Verification items for the finished model (mm, model axes). Face numbers are marked on the shaded views. A direction names the side the tool comes from. Give positions to 0.01 mm unless a question says otherwise; leave off trailing zeros. Write each loop counter-clockwise with the first axis right and the second up, starting at its lowest first coordinate (ties: lowest second). Pieces come first, ordered by that corner, then holes. Notation, with made-up numbers: (80, -31) - (103, -31) arc R22 ccw to (103, -18) - close; hole circle Ø2 at (-8, -28.5). An arc over 180 degrees is marked (long way). Answer as a JSON object with one key per item and string values. Group by question number.
Item 1: Go/stop test with flat-tipped pins: pin 1 (3.5 mm diameter, centred on x = 54.05, y = -5.05, fed in from +Z); pin 2 (10.5 mm diameter, centred on y = -10, z = 16.43, fed in from -X); pin 3 (1.6 mm diameter, centred on y = -3, z = 16.43, fed in from -X); pin 4 (1.2 mm diameter, centred on y = -17.5, z = 8.93, fed in from +X). Record where each tip stops, or that it passes through.
Item 2: Scan lines: line 1 along Y through (x, z) = (44.15, -0.65); line 2 along X through (y, z) = (-1.75, 16.5); line 3 along Z through (x, y) = (72.15, -17.5). Record each from-to range of solid material in increasing order. Write a range as [from, to].
Item 3: Draft check along X on the marked faces 1, 2 and 3. Enter one of: +X half, -X half, draft (parallel to the pull), parting line (faces both ways), or undercut.
Item 4: Sectioned sample at B-B, the plane z = 11. Record the boundary of the cut face in (x, y), and give its area (3 significant figures).
Item 5: Sectioned sample at A-A, the plane x = 54.05. Record the boundary of the cut face in (y, z), and give its area (3 significant figures).
Item 6: Sectioned sample at C-C, the plane y = -5.05. Record the boundary of the cut face in (x, z), and give its area (3 significant figures).
Item 7: Tool access check on the marked faces 4 and 5. Record the directions out of +Z, -Z, +X, -X, +Y, -Y that give a thin tool (end or side, any length) a straight path to the whole face; none if there is none.
Item 8: Sectioned sample at D-D, the plane y = -8. Record the boundary of the cut face in (x, z).
```python
from build123d import *

# Parameters (mm, degrees)
IZIM1_R                      = 4
IZIM1_R_2                    = 1
IZIM1_R_3                    = 3
IZIM1_R_4                    = 1.5
TABAN_FLAN_2_DEPTH           = 2
IZGIDEN_START                = -1
IZGIDEN_B_KME2_OUTLINE_W     = 20
IZGIDEN_B_KME2_OUTLINE_H     = 2
IZGIDEN_B_KME2_DEPTH         = 26.570796327
IZGIDEN_START_2              = 72.629203673
IZGIDEN_B_KME2_2_OUTLINE_W   = 20
IZGIDEN_B_KME2_2_OUTLINE_H   = 2
IZGIDEN_B_KME2_2_DEPTH       = 25.570796327
IZGIDEN_START_3              = 25.570796327
IZGIDEN_B_KME2_3_OUTLINE_R   = 1
IZGIDEN_B_KME2_3_OUTLINE_R_2 = 4
IZGIDEN_B_KME2_3_DEPTH       = 3
IZGIDEN_START_4              = 69.629203673
IZGIDEN_B_KME2_4_OUTLINE_R   = 1
IZGIDEN_B_KME2_4_OUTLINE_R_2 = 4
IZGIDEN_B_KME2_4_DEPTH       = 3
IZGIDEN_START_5              = 70.629203673
IZGIDEN_B_KME2_5_OUTLINE_R   = 1
IZGIDEN_B_KME2_5_DEPTH       = 2
IZGIDEN_B_KME2_6_OUTLINE_R   = 1
IZGIDEN_B_KME2_6_DEPTH       = 2
IZGIDEN_START_6              = -21
IZGIDEN_B_KME2_7_DEPTH       = 22


with BuildPart() as part:
    # Taban-Flanş2: sheet metal written as solids
    # Çizim1 → Taban-Flanş2 (new body)
    with BuildSketch(Plane.XY):
        with BuildLine():
            Line((98.2, -3), (98.2, -17))
            ThreePointArc((98.2, -17), (97.321320344, -19.121320344), (95.2, -20))
            Line((95.2, -20), (10, -20))
            ThreePointArc((10, -20), (0, -10), (10, 0))
            Line((10, 0), (95.2, 0))
            ThreePointArc((95.2, 0), (97.321320344, -0.878679656), (98.2, -3))
        make_face()
        with Locations((10, -10)):
            Circle(IZIM1_R, mode=Mode.SUBTRACT)
        with Locations((10, -17)):
            Circle(IZIM1_R_2, mode=Mode.SUBTRACT)
        with Locations((3, -10)):
            Circle(IZIM1_R_2, mode=Mode.SUBTRACT)
        with Locations((10, -3)):
            Circle(IZIM1_R_2, mode=Mode.SUBTRACT)
        with Locations((17, -10)):
            Circle(IZIM1_R_2, mode=Mode.SUBTRACT)
        with Locations((88.2, -10)):
            Circle(IZIM1_R, mode=Mode.SUBTRACT)
        with Locations((80.7, -2.5)):
            Circle(IZIM1_R_2, mode=Mode.SUBTRACT)
        with Locations((95.7, -2.5)):
            Circle(IZIM1_R_2, mode=Mode.SUBTRACT)
        with Locations((95.7, -17.5)):
            Circle(IZIM1_R_2, mode=Mode.SUBTRACT)
        with Locations((80.7, -17.5)):
            Circle(IZIM1_R_2, mode=Mode.SUBTRACT)
        with Locations((49.1, -10)):
            Circle(IZIM1_R_3, mode=Mode.SUBTRACT)
        with Locations((54.05, -5.05)):
            Circle(IZIM1_R_4, mode=Mode.SUBTRACT)
        with Locations((44.15, -5.05)):
            Circle(IZIM1_R_4, mode=Mode.SUBTRACT)
        with Locations((44.15, -14.95)):
            Circle(IZIM1_R_4, mode=Mode.SUBTRACT)
        with Locations((54.05, -14.95)):
            Circle(IZIM1_R_4, mode=Mode.SUBTRACT)
    extrude(amount=-TABAN_FLAN_2_DEPTH)

    # Çizgiden Bükme2: read off the stored shape, not the designer's step
    # Çizgiden Bükme2 outline → Çizgiden Bükme2 (cut)
    with BuildSketch(Plane.YZ.offset(IZGIDEN_START)):
        with Locations((-10, -1)):
            Rectangle(IZGIDEN_B_KME2_OUTLINE_W, IZGIDEN_B_KME2_OUTLINE_H)
    extrude(amount=IZGIDEN_B_KME2_DEPTH, mode=Mode.SUBTRACT)

    # izgiden B_kme2 2 outline → izgiden B_kme2 2 (cut)
    with BuildSketch(Plane.YZ.offset(IZGIDEN_START_2)):
        with Locations((-10, -1)):
            Rectangle(IZGIDEN_B_KME2_2_OUTLINE_W, IZGIDEN_B_KME2_2_OUTLINE_H)
    extrude(amount=IZGIDEN_B_KME2_2_DEPTH, mode=Mode.SUBTRACT)

    # izgiden B_kme2 3 outline → izgiden B_kme2 3 (add)
    with BuildSketch(Plane.YZ.offset(IZGIDEN_START_3)):
        with BuildLine():
            Line((-20, 0), (0, 0))
            Line((0, 0), (0, 16.429203673))
            ThreePointArc((0, 16.429203673), (-0.620384974, 19.896597791), (-2.404564394, 22.933768067))
            ThreePointArc((-2.404564394, 22.933768067), (-3.207106781, 23.222096892), (-3.495435606, 24.024639279))
            ThreePointArc((-3.495435606, 24.024639279), (-10, 26.429203673), (-16.504564394, 24.024639279))
            ThreePointArc((-16.504564394, 24.024639279), (-16.792893219, 23.222096892), (-17.595435606, 22.933768067))
            ThreePointArc((-17.595435606, 22.933768067), (-19.379615026, 19.896597791), (-20, 16.429203673))
            Line((-20, 16.429203673), (-20, 0))
        make_face()
        with Locations((-17.5, 8.929203673)):
            Circle(IZGIDEN_B_KME2_3_OUTLINE_R, mode=Mode.SUBTRACT)
        with Locations((-10, 9.429203673)):
            Circle(IZGIDEN_B_KME2_3_OUTLINE_R, mode=Mode.SUBTRACT)
        with Locations((-2.5, 8.929203673)):
            Circle(IZGIDEN_B_KME2_3_OUTLINE_R, mode=Mode.SUBTRACT)
        with Locations((-17, 16.429203673)):
            Circle(IZGIDEN_B_KME2_3_OUTLINE_R, mode=Mode.SUBTRACT)
        with Locations((-10, 16.429203673)):
            Circle(IZGIDEN_B_KME2_3_OUTLINE_R_2, mode=Mode.SUBTRACT)
        with Locations((-3, 16.429203673)):
            Circle(IZGIDEN_B_KME2_3_OUTLINE_R, mode=Mode.SUBTRACT)
        with Locations((-10, 23.429203673)):
            Circle(IZGIDEN_B_KME2_3_OUTLINE_R, mode=Mode.SUBTRACT)
    extrude(amount=IZGIDEN_B_KME2_3_DEPTH)

    # izgiden B_kme2 4 outline → izgiden B_kme2 4 (add)
    with BuildSketch(Plane.YZ.offset(IZGIDEN_START_4)):
        with BuildLine():
            Line((-20, 0), (0, 0))
            Line((0, 0), (0, 16.429203673))
            ThreePointArc((0, 16.429203673), (-0.620384974, 19.896597791), (-2.404564394, 22.933768067))
            ThreePointArc((-2.404564394, 22.933768067), (-3.207106781, 23.222096892), (-3.495435606, 24.024639279))
            ThreePointArc((-3.495435606, 24.024639279), (-10, 26.429203673), (-16.504564394, 24.024639279))
            ThreePointArc((-16.504564394, 24.024639279), (-16.792893219, 23.222096892), (-17.595435606, 22.933768067))
            ThreePointArc((-17.595435606, 22.933768067), (-19.379615026, 19.896597791), (-20, 16.429203673))
            Line((-20, 16.429203673), (-20, 0))
        make_face()
        with Locations((-17.5, 8.929203673)):
            Circle(IZGIDEN_B_KME2_4_OUTLINE_R, mode=Mode.SUBTRACT)
        with Locations((-10, 9.429203673)):
            Circle(IZGIDEN_B_KME2_4_OUTLINE_R, mode=Mode.SUBTRACT)
        with Locations((-2.5, 8.929203673)):
            Circle(IZGIDEN_B_KME2_4_OUTLINE_R, mode=Mode.SUBTRACT)
        with Locations((-17, 16.429203673)):
            Circle(IZGIDEN_B_KME2_4_OUTLINE_R, mode=Mode.SUBTRACT)
        with Locations((-10, 16.429203673)):
            Circle(IZGIDEN_B_KME2_4_OUTLINE_R_2, mode=Mode.SUBTRACT)
        with Locations((-3, 16.429203673)):
            Circle(IZGIDEN_B_KME2_4_OUTLINE_R, mode=Mode.SUBTRACT)
        with Locations((-10, 23.429203673)):
            Circle(IZGIDEN_B_KME2_4_OUTLINE_R, mode=Mode.SUBTRACT)
    extrude(amount=IZGIDEN_B_KME2_4_DEPTH)

    # izgiden B_kme2 5 outline → izgiden B_kme2 5 (add)
    with BuildSketch(Plane.YZ.offset(IZGIDEN_START_5)):
        with BuildLine():
            ThreePointArc((-2.404564394, 22.933768067), (-0.620384974, 19.896597791), (0, 16.429203673))
            Line((0, 16.429203673), (0, 23.429203673))
            ThreePointArc((0, 23.429203673), (-0.878679656, 25.550524017), (-3, 26.429203673))
            Line((-3, 26.429203673), (-10, 26.429203673))
            ThreePointArc((-10, 26.429203673), (-6.532605882, 25.808818699), (-3.495435606, 24.024639279))
            ThreePointArc((-3.495435606, 24.024639279), (-1.792893219, 24.636310454), (-2.404564394, 22.933768067))
        make_face()
        with BuildLine():
            Line((-20, 23.429203673), (-20, 16.429203673))
            ThreePointArc((-20, 16.429203673), (-19.379615026, 19.896597791), (-17.595435606, 22.933768067))
            ThreePointArc((-17.595435606, 22.933768067), (-18.207106781, 24.636310454), (-16.504564394, 24.024639279))
            ThreePointArc((-16.504564394, 24.024639279), (-13.467394118, 25.808818699), (-10, 26.429203673))
            Line((-10, 26.429203673), (-17, 26.429203673))
            ThreePointArc((-17, 26.429203673), (-19.121320344, 25.550524017), (-20, 23.429203673))
        make_face()
        with Locations((-17, 16.429203673)):
            Circle(IZGIDEN_B_KME2_5_OUTLINE_R)
        with Locations((-10, 23.429203673)):
            Circle(IZGIDEN_B_KME2_5_OUTLINE_R)
        with Locations((-3, 16.429203673)):
            Circle(IZGIDEN_B_KME2_5_OUTLINE_R)
        with Locations((-10, 9.429203673)):
            Circle(IZGIDEN_B_KME2_5_OUTLINE_R)
    extrude(amount=IZGIDEN_B_KME2_5_DEPTH)

    # izgiden B_kme2 6 outline → izgiden B_kme2 6 (add)
    with BuildSketch(Plane.YZ.offset(IZGIDEN_START_3)):
        with BuildLine():
            ThreePointArc((-3.495435606, 24.024639279), (-3.207106781, 23.222096892), (-2.404564394, 22.933768067))
            ThreePointArc((-2.404564394, 22.933768067), (-2.928932188, 23.500271485), (-3.495435606, 24.024639279))
        make_face()
        with BuildLine():
            ThreePointArc((-16.504564394, 24.024639279), (-17.071067812, 23.500271485), (-17.595435606, 22.933768067))
            ThreePointArc((-17.595435606, 22.933768067), (-16.792893219, 23.222096892), (-16.504564394, 24.024639279))
        make_face()
        with Locations((-2.5, 8.929203673)):
            Circle(IZGIDEN_B_KME2_6_OUTLINE_R)
        with Locations((-17.5, 8.929203673)):
            Circle(IZGIDEN_B_KME2_6_OUTLINE_R)
    extrude(amount=IZGIDEN_B_KME2_6_DEPTH)

    # izgiden B_kme2 7 outline → izgiden B_kme2 7 (cut)
    with BuildSketch(Plane(origin=(0, 0, 0), x_dir=(1, 0, 0), z_dir=(0, 1, 0)).offset(IZGIDEN_START_6)):
        with BuildLine():
            ThreePointArc((25.570796327, -1), (26.449475983, 1.121320344), (28.570796327, 2))
            Line((28.570796327, 2), (25.570796327, 1.999999978))
            Line((25.570796327, 1.999999978), (25.570796327, -1))
        make_face()
        with BuildLine():
            Line((72.629203673, 1.999999978), (69.629203673, 2))
            ThreePointArc((69.629203673, 2), (71.750524017, 1.121320344), (72.629203673, -1))
            Line((72.629203673, -1), (72.629203673, 1.999999978))
        make_face()
        with BuildLine():
            Line((27.570796327, -1), (27.570796327, -28))
            Line((27.570796327, -28), (28.570796327, -28))
            Line((28.570796327, -28), (28.570796327, 0))
            ThreePointArc((28.570796327, 0), (27.863689546, -0.292893219), (27.570796327, -1))
        make_face()
        with BuildLine():
            Line((69.629203673, -28), (70.629203673, -28))
            Line((70.629203673, -28), (70.629203673, -1))
            ThreePointArc((70.629203673, -1), (70.336310454, -0.292893219), (69.629203673, 0))
            Line((69.629203673, 0), (69.629203673, -28))
        make_face()
    extrude(amount=IZGIDEN_B_KME2_7_DEPTH, mode=Mode.SUBTRACT)


solid = part.part
```
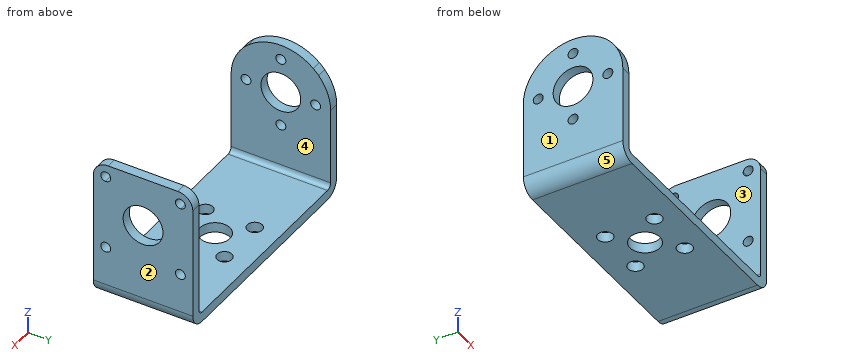
Geometry check:
{
 "1": {"pin 1": "z = 0", "pin 2": "x = 25.57", "pin 3": "x = 70.63", "pin 4": "x = 27.57"},
 "2": {"line 1": "[-20, -16.45], [-13.45, -6.55], [-3.55, 0]", "line 2": "[25.57, 27.57], [70.63, 72.63]", "line 3": "[-0.63, 7.93], [9.93, 22.93], [24.93, 26.39]"},
 "3": {"face 1": "-X half", "face 2": "+X half", "face 3": "undercut"},
 "4": {"outline": "(25.57, -20) - (27.57, -20) - (27.57, 0) - (25.57, 0) - close; (70.63, -20) - (72.63, -20) - (72.63, 0) - (70.63, 0) - close", "area": "80.0 mm^2"},
 "5": {"outline": "(-20, -2) - (-16.45, -2) - (-16.45, 0) - (-20, 0) - close; (-13.45, -2) - (-6.55, -2) - (-6.55, 0) - (-13.45, 0) - close; (-3.55, -2) - (0, -2) - (0, 0) - (-3.55, 0) - close", "area": "28.0 mm^2"},
 "6": {"outline": "(25.57, 1) arc R3 ccw to (28.57, -2) - (42.65, -2) - (42.65, 0) - (28.57, 0) arc R1 cw to (27.57, 1) - (27.57, 25.12) - (25.57, 25.12) - close; (45.65, -2) - (52.55, -2) - (52.55, 0) - (45.65, 0) - close; (55.55, -2) - (69.63, -2) arc R3 ccw to (72.63, 1) - (72.63, 26.43) - (70.63, 26.43) - (70.63, 1) arc R1 cw to (69.63, 0) - (55.55, 0) - close", "area": "182 mm^2"},
 "7": {"face 4": "+Z, +Y, -Y", "face 5": "-Z, -X, +Y, -Y"},
 "8": {"outline": "(25.57, 1) arc R3 ccw to (28.57, -2) - (46.86, -2) - (46.86, 0) - (28.57, 0) arc R1 cw to (27.57, 1) - (27.57, 12.97) - (25.57, 12.97) - close; (25.57, 19.89) - (27.57, 19.89) - (27.57, 26.23) - (25.57, 26.23) - close; (51.34, -2) - (69.63, -2) arc R3 ccw to (72.63, 1) - (72.63, 12.97) - (70.63, 12.97) - (70.63, 1) arc R1 cw to (69.63, 0) - (51.34, 0) - close; (70.63, 19.89) - (72.63, 19.89) - (72.63, 26.43) - (70.63, 26.43) - close"}
}
